Design review of the part shown in the three views and the two pictorial views. Dimensions are in mm from the part's minimum x, y and z. Give positions to 0.01 mm unless a question says otherwise; leave off trailing zeros. Loops run counter-clockwise (first coordinate to the right, second up) from the corner with the lowest first, then second, coordinate; pieces in that order, holes last. Notation, with made-up numbers: (43.25, -7) -> (77.25, -7) arc R38 ccw to (77.25, 31) -> close; hole circle Ø8 at (-7.75, 30.25). An arc over 180 degrees is marked (long way). One line per question, with ' | ' between items. Start each with the question number.
(1) Insertion check: P1, Ø3, axis at y = 2.5, z = 51, coming from the -X side; P2, Ø3.5, axis at x = 75, z = 65, coming from the +Y side. Each pin has a flat end and moves straight along its axis. Give the tip position at first contact, or say it passes through.
(2) Wall thickness on probe 1 along X at (y, z) = (2.9, 65); probe 2 along Z at (x, y) = (10, 2.7); probe 3 along X at (y, z) = (3.9, 55.5): over which ranges is each line inside the solid? List them lowest first.
(3) Consider section A-A (z = 65). Write out the cut boundary in (x, y), and give its area (3 significant figures).
(4) Consider section C-C (y = 2.9). Give the number of separate pieces and of enclosed holes in the cut face, and give its area (3 significant figures).
(5) Consider section D-D (z = 43.5). Write out the cut boundary in (x, y), and give its area (3 significant figures).
(6) Consider section B-B (x = 85). Write out the cut boundary in (y, z), and give its area (3 significant figures).
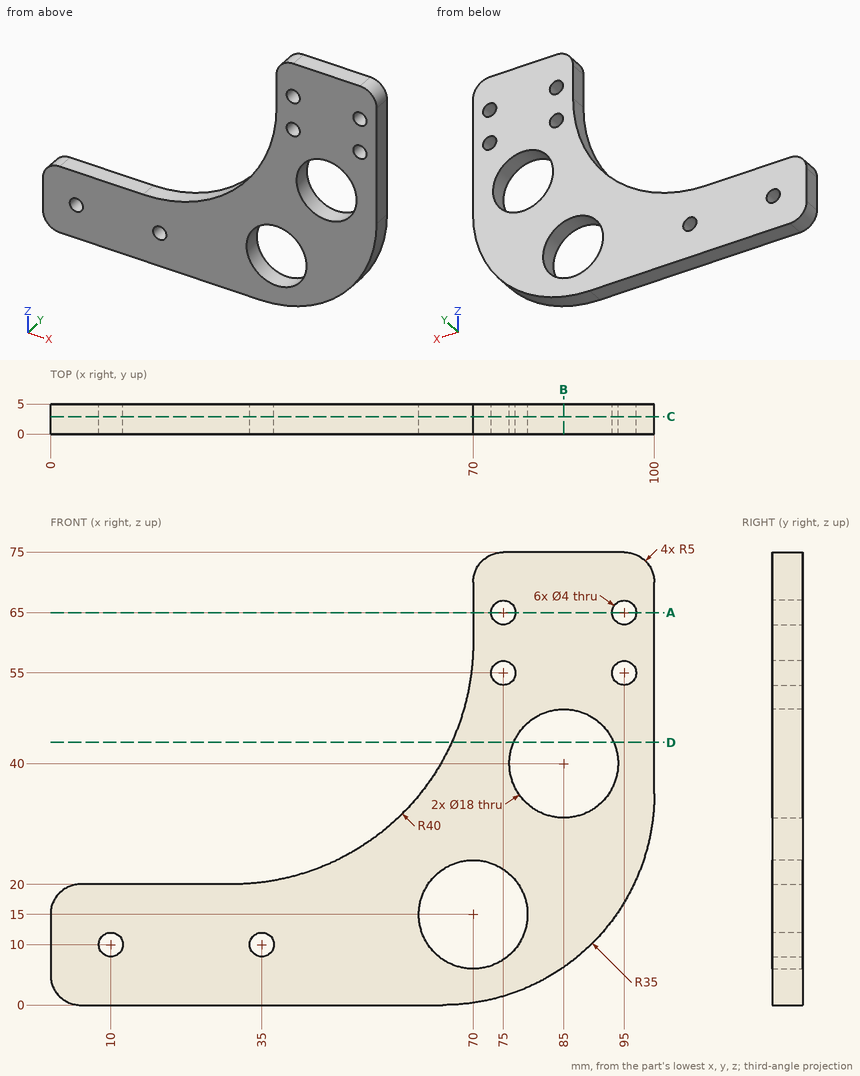
A:
1) P1: stops at x = 68.6 | P2: passes through
2) probe 1: x = 70 to 73, 77 to 93, 97 to 100 | probe 2: z = 0 to 8, 12 to 20 | probe 3: x = 69.75 to 73.06, 76.94 to 93.06, 96.94 to 100
3) outline: (70, 0) -> (73, 0) -> (73, 5) -> (70, 5) -> close; (77, 0) -> (93, 0) -> (93, 5) -> (77, 5) -> close; (97, 0) -> (100, 0) -> (100, 5) -> (97, 5) -> close | area: 110 mm^2
4) separate pieces: 1 | enclosed holes: 8 | area: 3,120 mm^2
5) outline: (66.44, 0) -> (76.71, 0) -> (76.71, 5) -> (66.44, 5) -> close; (93.29, 0) -> (100, 0) -> (100, 5) -> (93.29, 5) -> close | area: 84.9 mm^2
6) outline: (0, 6.28) -> (5, 6.28) -> (5, 31) -> (0, 31) -> close; (0, 49) -> (5, 49) -> (5, 75) -> (0, 75) -> close | area: 254 mm^2
